Autodesk Inventor part; units mm, degrees
ref_plane "YZ Plane" through (0, 0, 0) normal (1, 0, 0) x (0, 1, 0)
ref_plane "XZ Plane" through (0, 0, 0) normal (0, 1, 0) x (-1, 0, 0)
ref_plane "XY Plane" through (0, 0, 0) normal (0, 0, 1) x (1, 0, 0)
sketch "Boceto1" plane through (0, 0, 0) normal (0, 1, 0) x (-1, 0, 0)
  line L0 (47.5, 5) -> (-47.5, 5)
  line L1 (-47.5, 5) -> (-47.5, -5)
  line L2 (-47.5, -5) -> (47.5, -5)
  line L3 (47.5, -5) -> (47.5, 5)
  line L4 (47.5, 5) -> (-47.5, -5) construction
  line L5 (-47.5, 5) -> (47.5, -5) construction
  point P0 (0, 0)
  dimension "d0" = 95
  dimension "d1" = 10
extrude "Extrusión1" add sketch "Boceto1" along normal blind 3
sketch "Boceto2" plane through (0, 3, 0) normal (0, 1, 0) x (1, 0, 0)
  circle A0 centre (40.5, 0) radius 1.5
  line L0 (47.5, 5) -> (-47.5, 5)
  line L1 (47.5, -5) -> (47.5, 5)
  point P0 (0, 0)
  point P1 (47.5, 0)
  point P2 (47.5, 0)
  dimension "d4" = 3
  dimension "d5" = 5
  dimension "d7" = 7
extrude "Extrusión2" cut sketch "Boceto2" against normal blind 3
fillet "Empalme1" radius 2 1 edges at (-47.5, 1.5, 5)
fillet "Empalme2" radius 2 1 edges at (-47.5, 1.5, -5)
fillet "Empalme3" radius 2 1 edges at (47.5, 1.5, 5)
fillet "Empalme4" radius 2 1 edges at (47.5, 1.5, -5)
sketch "Boceto3" plane through (0, 3, 0) normal (0, 1, 0) x (1, 0, 0)
  line L0 (-47.5, 3) -> (-47.5, -3)
  circle A0 centre (-47.5, 0) radius 30
  line L1 (-47.5, 0) -> (-17.5, 0) construction
  line L2 (-47.5, 0) -> (-17.5, 0) construction
  point P0 (0, 0)
  dimension "d14" = 60
extrude "Extrusión3" add sketch "Boceto3" against normal blind 3
sketch "Boceto4" plane through (0, 3, 0) normal (0, 1, 0) x (1, 0, 0)
  arc A0 (-17.9196, 5) -> (-17.9196, -5) centre (-47.5, 0) ccw
  line L0 (-68.7649, 21.0578) -> (-8.8386, 21.0578) construction
  line L1 (-47.5, 0) -> (-26.4422, 21.0578)
  line L2 (-47.5, 0) -> (-17.7197, 0) construction
  line L3 (-47.5, 0) -> (-17.7197, 0) construction
  line L4 (-47.5, 0) -> (-68.7132, -21.2132)
  line L5 (-69.7473, 20.126) -> (-9.853, 20.126) construction
  line L6 (-59.6555, 10.0342) -> (-39.9443, -9.677)
  line L7 (-54.1333, 8.7547) -> (-36.886, -8.4927)
  line L8 (-59.6555, 10.0342) -> (-69.7473, 20.126)
  line L9 (-54.1333, 8.7547) -> (-67.626, 22.2473)
  line L10 (-36.886, -8.4927) -> (-25.2527, -20.126)
  line L11 (-39.9443, -9.677) -> (-27.374, -22.2473)
  line L12 (-69.7473, -20.126) -> (-27.374, 22.2473)
  line L13 (-25.2527, 20.126) -> (-67.626, -22.2473)
  circle A1 centre (-47.5, 0) radius 25
  point P0 (0, 0)
  point P1 (-64.0852, -18.7065)
  point P2 (-30.9148, -18.7065)
  point P3 (-47.5, -2.1213)
  point P4 (-28.7935, -16.5852)
  point P5 (-28.7935, 16.5852)
  point P6 (-45.3787, 0)
  point P7 (-30.9148, 18.7065)
  point P8 (-64.0852, 18.7065)
  point P9 (-47.5, 2.1213)
  point P10 (-66.2065, 16.5852)
  point P11 (-66.2065, -16.5852)
  point P12 (-49.6213, 0)
  dimension "d20" = 45
  dimension "d23" = 3
  dimension "d32" = 3
  dimension "d33" = 1.5
  dimension "d34" = 50
extrude "Extrusión4" cut sketch "Boceto4" against normal blind 3 contours A1 L10 L7 L13 | L12 L7 L9 A1 | L6 L11 A1 L13 | L8 L6 L12 A1
properties part number "Brazo_Servo"
Read the model definition and answer for the solid it produces. Units are mm, in the model's axes. A direction names the side the tool comes from. Round coordinates to 2 decimals unless told otherwise and drop trailing zeros. Write each loop counter-clockwise with the first axis right and the second up, starting at its lowest first coordinate (ties: lowest second). Pieces come first, ordered by that corner, then holes. Notation, with made-up numbers: (85.5, -24) - (126.5, -24) arc R12 ccw to (126.5, -8) - close; hole circle Ø9 at (65, 78.25). An arc over 180 degrees is marked (long way). Use a Markdown table: item, result.
(1) The part is cut by section B-B (z = -15). Write down the section's boundary in (x, y), then the cut area to 3 significant figures.
Reported:
| item | result |
|---|---|
| outline | (-73.48, 0) - (-67.5, 0) - (-67.5, 3) - (-73.48, 3) - close; (-64.62, 0) - (-60.38, 0) - (-60.38, 3) - (-64.62, 3) - close; (-34.62, 0) - (-30.38, 0) - (-30.38, 3) - (-34.62, 3) - close; (-27.5, 0) - (-21.52, 0) - (-21.52, 3) - (-27.5, 3) - close |
| area | 61.3 mm2 |
(2) The mould has two halves that part along Z. Classify faces 6 (the flat face through (-19, 3, 0)), 7 (the cylindrical face through (-77.474, 1.521, -1.249)), 8 (the cylindrical face through (-22.5, 1.5, 0.3)): released by +Z, released by -Z, zero draft, split by the parting line, or undercut.
Reported:
| item | result |
|---|---|
| face 6 | zero draft |
| face 7 | split by the parting line |
| face 8 | undercut |
(3) The part is cut by section D-D (x = -52.5). Write down the section's boundary in (y, z), then the cut area to 3 significant figures.
Reported:
| item | result |
|---|---|
| outline | (0, -29.58) - (3, -29.58) - (3, -24.49) - (0, -24.49) - close; (0, -7.12) - (3, -7.12) - (3, -2.88) - (0, -2.88) - close; (0, 2.88) - (3, 2.88) - (3, 7.12) - (0, 7.12) - close; (0, 24.49) - (3, 24.49) - (3, 29.58) - (0, 29.58) - close |
| area | 56.0 mm2 |
(4) Each of these flat-tipped pins is pushed along its axis until it touches: pin 1 Ø0.9 at (x, y) = (14, 1.5) entering from +Z; pin 2 Ø0.9 at (x, y) = (-0.5, 1.5) entering from -Z. Where does it stop, or does it pass through?
Reported:
| item | result |
|---|---|
| pin 1 | z = 5 |
| pin 2 | z = -5 |
(5) The part is cut by section C-C (z = 20.5). Write down the section's boundary in (x, y), then the cut area to 3 significant figures.
Reported:
| item | result |
|---|---|
| outline | (-69.4, 0) - (-61.81, 0) - (-61.81, 3) - (-69.4, 3) - close; (-33.19, 0) - (-25.6, 0) - (-25.6, 3) - (-33.19, 3) - close |
| area | 45.6 mm2 |
(6) Which of the six approach directions +Z, -Z, +X, -X, +Y, -Y give full straight-line access (tool end or side, diameter ignored) to faces 1 (the flat face through (13, 1, 5)), 2 (the flat face through (47.5, 1, 0)), 3 (the flat face through (14, 1, -5)), 4 (the flat face through (-55.68, 1.52, 10.3)), 5 (the flat face through (-19, 0, 0))?
Reported:
| item | result |
|---|---|
| face 1 | +Z, +X, +Y, -Y |
| face 2 | +Z, -Z, +X, +Y, -Y |
| face 3 | -Z, +X, +Y, -Y |
| face 4 | +Y, -Y |
| face 5 | +Z, -Z, +X, -X, -Y |
(7) Straight lines are drawn through the part: line 1 along X through (y, z) = (1.6, 0); line 2 along X through (y, z) = (2.45, 10); line 3 along Z through (x, y) = (-61, 2.4). For each, find the intervals that lie inside material, in ascending order. Write a range as [from, to].
Reported:
| item | result |
|---|---|
| line 1 | [-77.5, -72.5], [-49.62, -45.38], [-22.5, 39], [42, 47.5] |
| line 2 | [-75.78, -70.41], [-59.62, -55.38], [-39.62, -35.38], [-24.59, -19.22] |
| line 3 | [-26.79, -21.04], [-15.62, -11.38], [11.38, 15.62], [21.04, 26.79] |
(8) The part is cut by section A-A (x = 40.5). Write down the section's boundary in (y, z).
Reported:
| item | result |
|---|---|
| outline | (0, -5) - (3, -5) - (3, -1.5) - (0, -1.5) - close; (0, 1.5) - (3, 1.5) - (3, 5) - (0, 5) - close |
